from build123d import *

# Parameters (mm, degrees)
F1_DEPTH = 6.35


# Not quite as in the source:
# - a feature names something its author has since deleted; it is built from what else it names


with BuildPart() as f1:
    # F0 (on Right) → F1 (new body)
    with BuildSketch(Plane.YZ):
        with BuildLine():
            Line((10.1997445822, -25.9578457783), (10.1997445822, -51.0764221646))
            Line((10.1997445822, -51.0764221646), (22.8997445822, -51.0764221646))
            ThreePointArc((22.8997445822, -51.0764221646), (24.7978912955, -42.2422146629), (32.0898325185, -36.9061321742))
            Line((32.0898325185, -36.9061321742), (137.1997445822, -36.9061321742))
            Line((137.1997445822, -36.9061321742), (137.2000693373, -17.6021321769))
            Line((137.2000693373, -17.6021321769), (149.8997445822, 6.2824831575))
            Line((149.8997445822, 6.2824831575), (137.1997445822, 6.2824831575))
            Line((137.1997445822, 6.2824831575), (22.8997445822, 6.2824831575))
            Line((22.8997445822, 6.2824831575), (22.8997445822, -20.3278172679))
            ThreePointArc((22.8997445822, -20.3278172679), (17.3877746683, -25.0332272954), (10.1997445822, -25.9578457783))
        make_face()
    extrude(amount=F1_DEPTH)


solid = f1.part
CAD build for the part. Positions are in the model's coordinates, mm. A direction names the side the tool comes from. Give positions to 0.01 mm unless a question says otherwise; leave off trailing zeros. Order: outer loops, then holes, each group sorted by start corner. A loop starts at its lowest first (then second) coordinate and runs counter-clockwise, first axis right, second up. Notation, with made-up numbers: (22, 51.25) -> (60, 51.25) arc R12 cw to (60, 63.25) -> close; hole circle Ø8 at (-26, 3). An arc over 180 degrees is marked (long way). Return JSON: item names as keys, results as strings.
Q1. Mould opens along Z. For faces 1 (the face through (3.13, 17.48, -24.99)), 2 (the face through (3, 22.9, -7)), 3 (the face through (3.13, 24.73, -42.35)) say: pulls with the +Z half, pulls with the -Z half, needs draft (parallel to the pull), parting line crosses it, or undercut.
Working result:
{"face 1": "pulls with the +Z half", "face 2": "needs draft", "face 3": "undercut"}
Q2. Saw through at B-B (y = 55). Write the cut outline in (x, z), then the cut area to 3 significant figures.
Working result:
{"outline": "(0, -36.91) -> (6.35, -36.91) -> (6.35, 6.28) -> (0, 6.28) -> close", "area": "274 mm²"}
Q3. Saw through at C-C (z = 0). Write the cut outline in (x, y).
Working result:
{"outline": "(0, 22.9) -> (6.35, 22.9) -> (6.35, 146.56) -> (0, 146.56) -> close"}
Q4. Which spindle directions (+Z, -Z, +X, -X, +Y, -Y) get a long thin tool onto all of the face, cutting with end or side? Do faces 4 (the face through (3, 84, -36.906)), 5 (the face through (6.35, 79, -16)). Say none if no direction does.
Working result:
{"face 4": "-Z, +X, -X, +Y", "face 5": "+Z, -Z, +X, +Y, -Y"}
Q5. Flat gauge pins, fed straight in: pin 1 (1.5 mm diameter, centred on x = 1.5, y = 47, fed in from -Z); pin 2 (1.5 mm diameter, centred on x = 1.5, z = -10.5, fed in from +Y); pin 3 (3 mm diameter, centred on x = 2.5, z = -28.5, fed in from +Y). Where does each tip first touch, or does it go through?
Working result:
{"pin 1": "z = -36.91", "pin 2": "y = 141.38", "pin 3": "y = 137.2"}
Q6. Drill centre lines: line 1 (Z direction, x = 3.5, y = 63); line 2 (Y direction, x = 2.25, z = -18.5); line 3 (Y direction, x = 3, z = -30.5). Where is each one in solid material? Low to high.
Working result:
{"line 1": "-36.91 to 6.28", "line 2": "22.9 to 137.2", "line 3": "10.2 to 137.2"}
Q7. Saw through at A-A (x = 3.25). Write the cut outline in (y, z), then the cut area to 3 significant figures.
Working result:
{"outline": "(10.2, -51.08) -> (22.9, -51.08) arc R12.7 cw to (32.09, -36.91) -> (137.2, -36.91) -> (137.2, -17.6) -> (149.9, 6.28) -> (22.9, 6.28) -> (22.9, -20.33) arc R12.7 cw to (10.2, -25.96) -> close", "area": "5,450 mm²"}
